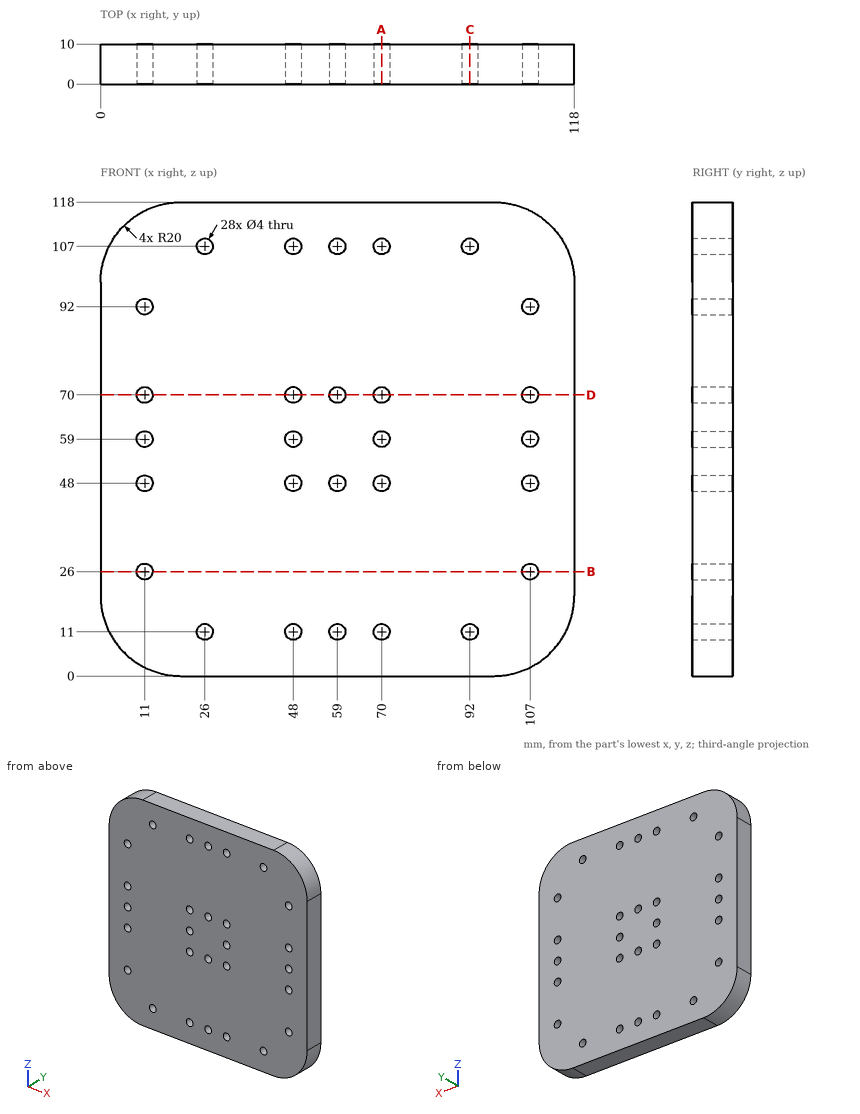
Design review of the part shown in the three views and the two pictorial views. Dimensions are in mm from the part's minimum x, y and z. Give positions to 0.01 mm unless a question says otherwise; leave off trailing zeros. Order: outer loops, then holes, each group sorted by start corner. A loop starts at its lowest first (then second) coordinate and runs counter-clockwise, first axis right, second up. Notation, with made-up numbers: (-2, 68) -> (21, 68) arc R28 cw to (21, 93) -> close; hole circle Ø11 at (62.25, -1.5). An arc over 180 degrees is marked (long way). Write each question's results on one line, items separated by ' | '. Start each with the question number.
Q1. Add section A-A on x = 70. Give the boundary of the cut face in (y, z).
Q2. For pin 1 (2 mm diameter, centred on x = 102, y = 5, fed in from -Z), flat-tipped, find the tip position at first contact; note if it passes through.
Q3. Add section C-C on x = 92. Give the boundary of the cut face in (y, z).
Q4. Add section D-D on z = 70. Give the boundary of the cut face in (x, y).
Q5. Add section B-B on z = 26. Give the boundary of the cut face in (x, y).
Q6. Wall thickness on L1, parallel to X at y = 4.5, z = 70; L2, parallel to Z at x = 69, y = 3.5; L3, parallel to X at y = 3.75, z = 107: over which ranges is each line inside the solid? List them lowest first. Write a range as from..to.
Found:
1) outline: (0, 0) -> (10, 0) -> (10, 9) -> (0, 9) -> close; (0, 13) -> (10, 13) -> (10, 46) -> (0, 46) -> close; (0, 50) -> (10, 50) -> (10, 57) -> (0, 57) -> close; (0, 61) -> (10, 61) -> (10, 68) -> (0, 68) -> close; (0, 72) -> (10, 72) -> (10, 105) -> (0, 105) -> close; (0, 109) -> (10, 109) -> (10, 118) -> (0, 118) -> close
2) pin 1: stops at z = 0.23
3) outline: (0, 0) -> (10, 0) -> (10, 9) -> (0, 9) -> close; (0, 13) -> (10, 13) -> (10, 105) -> (0, 105) -> close; (0, 109) -> (10, 109) -> (10, 118) -> (0, 118) -> close
4) outline: (0, 0) -> (9, 0) -> (9, 10) -> (0, 10) -> close; (13, 0) -> (46, 0) -> (46, 10) -> (13, 10) -> close; (50, 0) -> (57, 0) -> (57, 10) -> (50, 10) -> close; (61, 0) -> (68, 0) -> (68, 10) -> (61, 10) -> close; (72, 0) -> (105, 0) -> (105, 10) -> (72, 10) -> close; (109, 0) -> (118, 0) -> (118, 10) -> (109, 10) -> close
5) outline: (0, 0) -> (9, 0) -> (9, 10) -> (0, 10) -> close; (13, 0) -> (105, 0) -> (105, 10) -> (13, 10) -> close; (109, 0) -> (118, 0) -> (118, 10) -> (109, 10) -> close
6) L1: x = 0..9, 13..46, 50..57, 61..68, 72..105, 109..118 | L2: z = 0..9.27, 12.73..46.27, 49.73..57.27, 60.73..68.27, 71.73..105.27, 108.73..118 | L3: x = 2.14..24, 28..46, 50..57, 61..68, 72..90, 94..115.86
